```python
from build123d import *

# Parameters (mm, degrees)
SKETCH4_R          = 0.9921875
CUT_EXTRUDE1_DEPTH = 1.016
CUT_EXTRUDE2_START = -2.54
SKETCH3_R          = 0.9921875
CUT_EXTRUDE2_DEPTH = 2.54


with BuildPart() as part:
    # Sketch2 → Revolve1 (revolve)
    with BuildSketch(Plane(origin=(0, 0, 0), x_dir=(0, 0, -1), z_dir=(1, 0, 0)), mode=Mode.PRIVATE) as revolve1_sk:
        with BuildLine():
            Line((-1.27, 0.9921875), (-1.27, 0))
            Line((-1.27, 0), (19.05, 0))
            Line((19.05, 0), (22.225, 0))
            Line((22.225, 0), (22.225, 3.4925))
            Line((22.225, 3.4925), (19.05, 3.4925))
            Line((19.05, 3.4925), (19.05, 2.38125))
            Line((19.05, 2.38125), (0, 2.38125))
            Line((0, 2.38125), (0, 4.6228))
            Line((0, 4.6228), (-0.1778, 4.6228))
            ThreePointArc((-0.1778, 4.6228), (-0.991036966, 2.887856773), (-1.27, 0.9921875))
        make_face()
    revolve(revolve1_sk.sketch.rotate(Axis((0, 0, 7.600580616), (0, 0, 1)), 90), axis=Axis((0, 0, 7.600580616), (0, 0, 1)))

    # Sketch4 → Cut-Extrude1 (cut)
    with BuildSketch(Plane.XY.offset(1.27)):
        Circle(SKETCH4_R)
    extrude(amount=-CUT_EXTRUDE1_DEPTH, mode=Mode.SUBTRACT)

    # Sketch3 → Cut-Extrude2 (cut)
    with BuildSketch(Plane(origin=(0, 0, -22.225), x_dir=(-1, 0, 0), z_dir=(0, 0, -1)).offset(CUT_EXTRUDE2_START)):
        with Locations(Location((0, 0, 0), (0, 0, 180))):
            Circle(SKETCH3_R)
    extrude(amount=CUT_EXTRUDE2_DEPTH, mode=Mode.SUBTRACT)


solid = part.part
```
Read the model definition and answer for the solid it produces. Units are mm, in the model's axes. A direction names the side the tool comes from. Round coordinates to 2 decimals unless told otherwise and drop trailing zeros. Write each loop counter-clockwise with the first axis right and the second up, starting at its lowest first coordinate (ties: lowest second). Pieces come first, ordered by that corner, then holes. Notation, with made-up numbers: (75, 50) -> (108, 50) arc R28 ccw to (108, 70) -> close; hole circle Ø11 at (27, 62.5). An arc over 180 degrees is marked (long way). Answer in a Markdown table with one row per item. Add a question column.
1) Given P1, Ø1, axis at x = -2.5, z = -6.5, coming from the -Y side; P2, Ø1, axis at x = 1, z = -12.5, coming from the -Y side; P3, Ø3, axis at x = 2, z = -16, coming from the +Y side; P4, Ø3, axis at x = 0, y = 0, coming from the +Z side, each flat-ended and moving along its own axis, determine where each tip first touches the part or whether it passes through.
2) Which of the six approach directions +Z, -Z, +X, -X, +Y, -Y give full straight-line access (tool end or side, diameter ignored) to faces 1 (the face through (0, 0, 0.254)), 2 (the face through (0.516, 2.325, -9.392)), 3 (the face through (0, 0, -19.685)), 4 (the face through (1, 1, -22.225))?
3) Consider line 1 (Y direction, x = 0, z = -21.45); line 2 (Z direction, x = 0, y = -2.5) (3 decimals); line 3 (Z direction, x = -3.25, y = 0.5) (3 decimals). Determine where each line is inside the solid, lowest interval first.
4) Determine the mould class of faces 5 (the face through (0.455, -3.463, -20.615)), 6 (the face through (2, 2, 0)), 7 (the face through (-0.215, 0.969, -20.937)) for opening direction Y: pulls with the +Y half, pulls with the -Y half, needs draft (parallel to the pull), parting line crosses it, or undercut.
5) Find section A-A, the plane z = -2.75. Determine the outline of the cut face in (x, y), and give its area (3 significant figures).
Findings below:
| question | item | result |
|---|---|---|
| 1 | P1 | y = -1.29 |
| 1 | P2 | y = -2.33 |
| 1 | P3 | y = 2.33 |
| 1 | P4 | z = 1.27 |
| 2 | face 1 | +Z |
| 2 | face 2 | none |
| 2 | face 3 | -Z |
| 2 | face 4 | -Z, +X, -X, +Y, -Y |
| 3 | line 1 | -3.49 to -0.99, 0.99 to 3.49 |
| 3 | line 2 | -22.225 to -19.05, 0 to 1.095 |
| 3 | line 3 | -22.225 to -19.05, 0 to 0.856 |
| 4 | face 5 | parting line crosses it |
| 4 | face 6 | needs draft |
| 4 | face 7 | undercut |
| 5 | outline | circle Ø4.76 at (0, 0) |
| 5 | area | 17.8 mm² |
